For this review, use the dimensioned drawing (mm, ordinates from the lowest corner) and the shaded views. A direction names the side the tool comes from. Give positions to 0.01 mm unless a question says otherwise; leave off trailing zeros. Loops run counter-clockwise (first coordinate to the right, second up) from the corner with the lowest first, then second, coordinate; pieces in that order, holes last. Notation, with made-up numbers: (45, 74.5) -> (61, 74.5) arc R30 ccw to (61, 107.5) -> close; hole circle Ø10 at (-26.75, -6.5). An arc over 180 degrees is marked (long way). Use a Markdown table: item, result. Add a question column.
1. Add section A-A (y = 15). Count the separate pieces of the cut face and the enclosed holes in it, and give its area (3 significant figures).
2. Add section D-D (y = 4). State the section outline as (x, z) points, and give its area (3 significant figures).
3. For pin 1 Ø1.5 at (y, z) = (11.5, 38) entering from +X; pin 2 Ø3 at (x, y) = (76, 10) entering from -Z; pin 3 Ø10 at (x, y) = (6, 21) entering from +Z, all flat-tipped, find the tip position at first contact; note any pin that passes through.
4. To check wall thickness, follow line 1 (X direction, y = 21.5, z = 34); line 2 (Y direction, x = 10, z = 1.35); line 3 (Z direction, x = 54, y = 3.5). State the ranges of each line that lie inside material, in increasing order.
5. Add section C-C (z = 8.5). State the section outline as (x, y) points, and give its area (3 significant figures).
6. Add section B-B (x = 65). State the section outline as (y, z) points, and give its area (3 significant figures).
7. Draft analysis for pull direction X (two halves, no side actions). For the marked faces 4, 5 and 6, state which applies: pulls with the +X half, pulls with the -X half, needs draft (parallel to the pull), parting line crosses it, or undercut.
8. For the marked faces 1, 2 and 3, list the 3-axis set-ups (+Z, -Z, +X, -X, +Y, -Y) from which the entire face can be reached by the end or side of a thin tool; tool diameter is ignored.
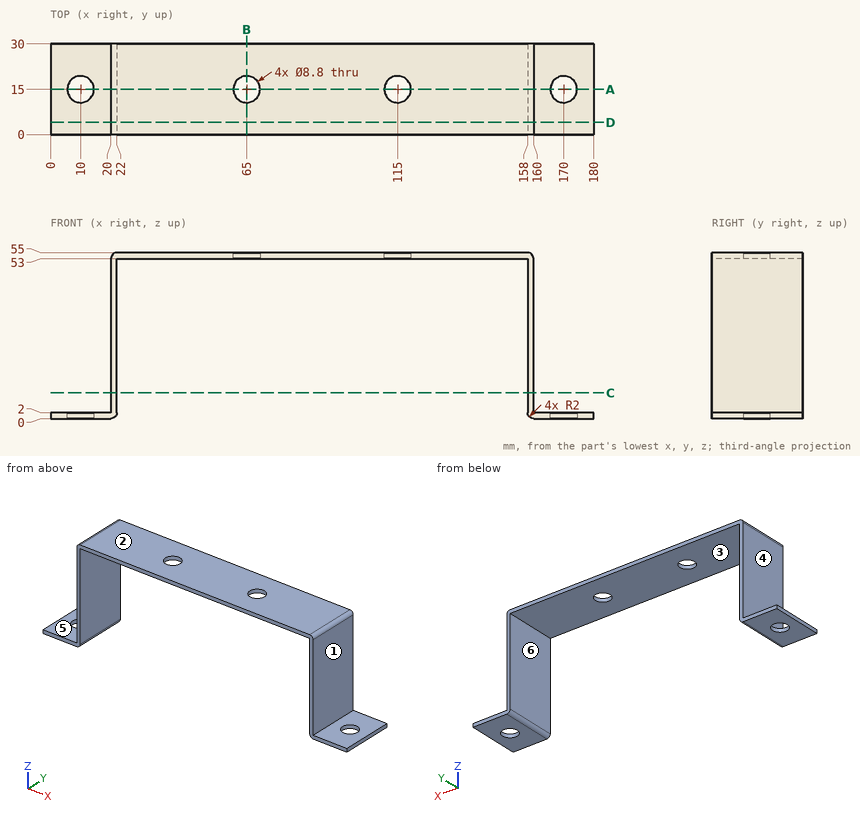
Taken from the geometry:
| question | item | result |
|---|---|---|
| 1 | separate pieces | 5 |
| 1 | enclosed holes | 0 |
| 1 | area | 498 mm^2 |
| 2 | outline | (0, 0) -> (20, 0) arc R2 ccw to (22, 2) -> (22, 53) -> (158, 53) -> (158, 2) arc R2 ccw to (160, 0) -> (180, 0) -> (180, 2) -> (160, 2) -> (160, 53) arc R2 ccw to (158, 55) -> (22, 55) arc R2 ccw to (20, 53) -> (20, 2) -> (0, 2) -> close |
| 2 | area | 569 mm^2 |
| 3 | pin 1 | stops at x = 160 |
| 3 | pin 2 | stops at z = 53 |
| 3 | pin 3 | stops at z = 2 |
| 4 | line 1 | x = 20 to 22, 158 to 160 |
| 4 | line 2 | y = 0 to 10.6, 19.4 to 30 |
| 4 | line 3 | z = 53 to 55 |
| 5 | outline | (20, 0) -> (22, 0) -> (22, 30) -> (20, 30) -> close; (158, 0) -> (160, 0) -> (160, 30) -> (158, 30) -> close |
| 5 | area | 120 mm^2 |
| 6 | outline | (0, 53) -> (10.6, 53) -> (10.6, 55) -> (0, 55) -> close; (19.4, 53) -> (30, 53) -> (30, 55) -> (19.4, 55) -> close |
| 6 | area | 42.4 mm^2 |
| 7 | face 4 | pulls with the -X half |
| 7 | face 5 | needs draft |
| 7 | face 6 | undercut |
| 8 | face 1 | +Z, +X, +Y, -Y |
| 8 | face 2 | +Z, +X, -X, +Y, -Y |
| 8 | face 3 | -Z, +Y, -Y |
